Source: three-view drawing plus pictorial views. Frame: mm from the lowest corner of the part. Coordinates: 2 decimals unless noted, no trailing zeros. Loops run counter-clockwise (first coordinate to the right, second up) from the corner with the lowest first, then second, coordinate; pieces in that order, holes last. Notation, with made-up numbers: (38.25, 81) - (47.25, 81) arc R25 cw to (47.25, 114) - close; hole circle Ø2 at (-4.75, 77.25). An arc over 180 degrees is marked (long way). Return JSON: item names as keys, results as strings.
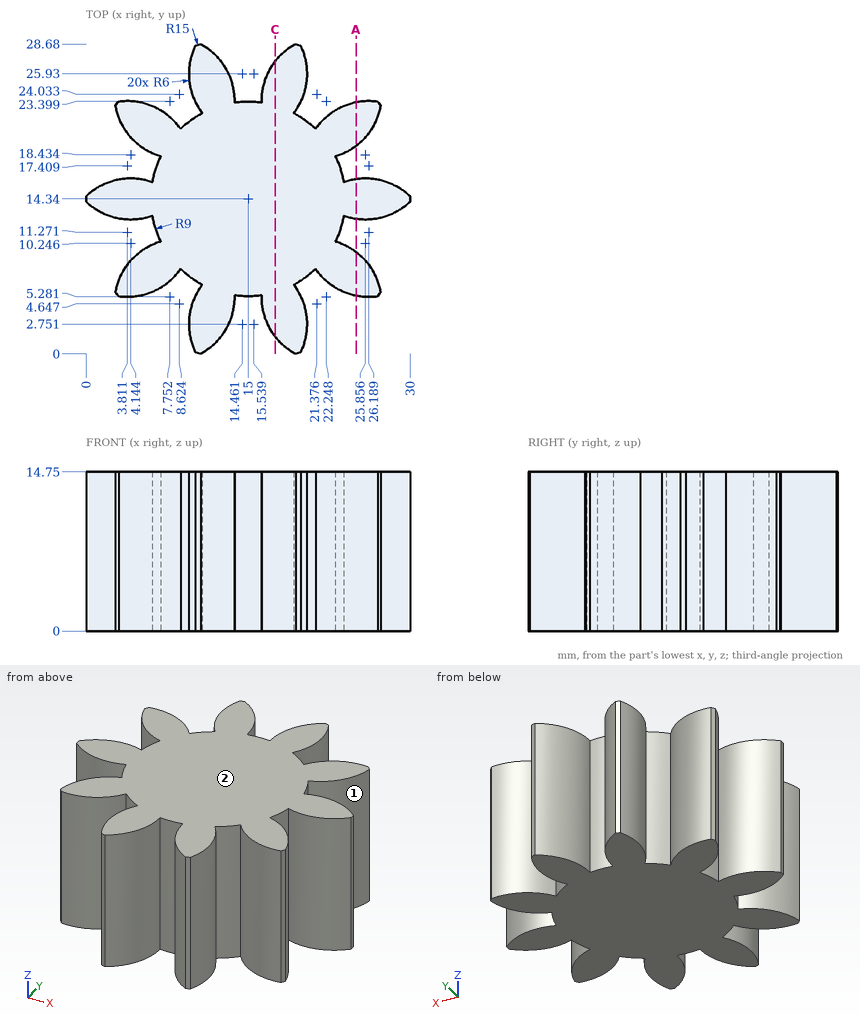
Item 1: Mould query, pull axis Y, two halves, no side actions, for the marked faces 1 and 2. Classes: +Y half, -Y half, draft (parallel to the pull), parting line (faces both ways), or undercut.
Worked out:
{"face 1": "undercut", "face 2": "draft"}
Item 2: Section query C-C, the plane x = 17.5. Return loops of the section in (y, z).
Worked out:
{"outline": "(1.61, 0) - (27.07, 0) - (27.07, 14.75) - (1.61, 14.75) - close"}
Item 3: Section query A-A, the plane x = 25. Count the separate pieces of the cut face and the enclosed holes in it.
Worked out:
{"separate pieces": "3", "enclosed holes": "0"}
Item 4: First-contact query: pin 1 Ø5 at (y, z) = (23, 2) entering from -X; pin 2 Ø1.5 at (y, z) = (14, 3) entering from +X; pin 3 Ø2 at (x, z) = (26.5, 5) entering from +Y. Flat tips, straight axial feed; report the tip coordinate or a pass-through.
Worked out:
{"pin 1": "x = 2.72", "pin 2": "x = 30", "pin 3": "y = 23.41"}
Item 5: Ray query, probe 1 along Y at (x, z) = (24.5, 14) (1 decimal); probe 2 along X at (y, z) = (21, 3.5) (1 decimal); probe 3 along Y at (x, z) = (4, 1.75) (1 decimal). Return the intervals inside material, ascending. Write a range as from..to.
Worked out:
{"probe 1": "5.5..9.8, 12.6..16.1, 18.9..23.2", "probe 2": "3.4..8.6, 8.9..21.1, 21.4..26.6", "probe 3": "5.3..8.5, 12.4..16.2, 20.2..23.4"}
